Build history of the part. All positions in model axes, mm. A direction names the side the tool comes from. Give positions to 0.01 mm unless a question says otherwise; leave off trailing zeros. Write each loop counter-clockwise with the first axis right and the second up, starting at its lowest first coordinate (ties: lowest second). Pieces come first, ordered by that corner, then holes. Notation, with made-up numbers: M -2,-10.75 L 40,-10.75 A16 ccw 40,1.25 Z; hole C 35.25,11 d7. An arc over 180 degrees is marked long. Return JSON: item names as keys, results as strings. Group by question number.
Q1. Tool access for faces 4 (the flat face through (-0.2, -5.4, 70)), 5 (the cylindrical face through (11.923, 3.755, 69.014)), 6 (the conical face through (4.663, 1.468, 60.388)): list every direction of +Z, -Z, +X, -X, +Y, -Y with a clear straight run to the whole face (end or side of a thin tool).
Q2. Wall check: probe 1 along Z at (x, y) = (10.25, -6); probe 2 along Z at (x, y) = (1.5, 9); probe 3 along X at (y, z) = (-2, 4.5). Give the ranges that are in metal, low to high.
Q3. Band-saw the part on A-A, the plane y = 0. Give the cut face in (x, z).
Q4. Pull direction Z, two halves, no side cores. Call faces 1 (the cylindrical face through (-1.08, -4.88, 74.93)), 2 (the cylindrical face through (-0.59, -4.46, 35.35)), 3 (the flat face through (0, 0, 80)): +Z half, -Z half, draft (parallel to the pull), parting line (faces both ways), or undercut.
Q5. Flat gauge pins, fed straight in: pin 1 Ø2 at (x, y) = (-1, 8) entering from +Z; pin 2 Ø5 at (y, z) = (7, 69.5) entering from -X; pin 3 Ø3 at (x, y) = (-3, 1.5) entering from -Z; pin 4 Ø3 at (y, z) = (3.5, 55.5) entering from -X. Where does each tip first touch, or does it go through?
Q6. Band-saw the part on C-C, the plane z = 33.5. Give the cut face in (x, y), then the cut area to 3 significant figures.
from build123d import *

# Parameters (mm, degrees)
F0_R      = 12.5
F1_DEPTH  = 2
F1_FACE_R = 12.5
F2_DEPTH  = 8
F2_TAPER  = 45
F3_DEPTH  = 25
F5_R      = 5
F6_DEPTH  = 10


with BuildPart() as f1:
    # F0 (on Top) → F1 (new body)
    with BuildSketch(Plane.XY):
        Circle(F0_R)
    extrude(amount=F1_DEPTH)

    # F1_face (on face) → F2 (join)
    with BuildSketch(Plane.XY.offset(2)):
        Circle(F1_FACE_R)
    extrude(amount=F2_DEPTH, taper=F2_TAPER)

    # F3 (add): a face of the model
    f3_faces = [f1.faces().sort_by_distance(p)[0] for p in [
        (0, 0, 10),
    ]]
    extrude(f3_faces, amount=F3_DEPTH)

    # F4: F1 across face


with BuildPart() as f1_1:
    add(f1.part)
    add(f1.part.mirror(Plane.XY.offset(35)))

    # F5 (on face) → F6 (join)
    with BuildSketch(Plane.XY.offset(70)):
        Circle(F5_R)
    extrude(amount=F6_DEPTH)


solid = f1_1.part
From the geometry:
{
 "1": {"face 4": "+Z", "face 5": "+Z, -Z", "face 6": "none"},
 "2": {"probe 1": "z = 0 to 2.62, 67.38 to 70", "probe 2": "z = 0 to 5.38, 64.62 to 70", "probe 3": "x = -9.8 to 9.8"},
 "3": {"outline": "M -12.5,0 L 12.5,0 L 12.5,2 L 4.5,10 L 4.5,60 L 12.5,68 L 12.5,70 L 5,70 L 5,80 L -5,80 L -5,70 L -12.5,70 L -12.5,68 L -4.5,60 L -4.5,10 L -12.5,2 Z"},
 "4": {"face 1": "draft", "face 2": "undercut", "face 3": "+Z half"},
 "5": {"pin 1": "stops at z = 70", "pin 2": "stops at x = -11.66", "pin 3": "stops at z = 0", "pin 4": "stops at x = -4.03"},
 "6": {"outline": "C 0,0 d9", "area": "63.6 mm^2"}
}
